Here's how the part is built. I have some questions about the finished solid (model axes, mm). Face numbers are marked on the shaded views. A direction names the side the tool comes from. Coordinates: 2 decimals unless noted, no trailing zeros. Loops run counter-clockwise (first coordinate to the right, second up) from the corner with the lowest first, then second, coordinate; pieces in that order, holes last. Notation, with made-up numbers: (65.25, 61) -> (96.25, 61) arc R26 cw to (96.25, 82) -> close; hole circle Ø7 at (-33.75, 87). An arc over 180 degrees is marked (long way). Use CSV: the item, a comma, the result in double quotes. Start each with the question number.
from build123d import *

# Parameters (mm, degrees)
BOSS_EXTRU_1_DEPTH      = 20
ENL_V_MAT_EXTRU_1_REACH = 77.705
ESQUISSE2_R             = 1.5
D_GAGEMENT_M31_D        = 3.4
D_GAGEMENT_M31_DEPTH    = 57.5
D_GAGEMENT_M31_TIP      = 1.021463052
CONG_1_R                = 10
CONG_2_R                = 5


with BuildPart() as part:
    # Esquisse1 → Boss.-Extru.1 (new body)
    with BuildSketch(Plane.XY):
        Polygon((0, 0), (4, 0), (4, 41), (53.5, 41), (53.5, 0), (57.5, 0), (57.5, 45), (0, 45), align=None)
    extrude(amount=BOSS_EXTRU_1_DEPTH)

    # Enlèv. mat.-Extru.1: up to this face of the body (flat: up to its plane)
    enl_v_mat_extru_1_end = Plane(part.part.faces().sort_by_distance((0, 22.5, 10))[0])
    # Esquisse2 → Enlèv. mat.-Extru.1 (cut, up to the picked face)
    with BuildSketch(Plane(origin=(57.5, 0, 0), x_dir=(0, 0, -1), z_dir=(1, 0, 0)), mode=Mode.PRIVATE) as enl_v_mat_extru_1_sk1:
        with Locations((-10, 5.5)):
            Circle(ESQUISSE2_R)
    enl_v_mat_extru_1_tool1 = split(extrude(enl_v_mat_extru_1_sk1.sketch, amount=-ENL_V_MAT_EXTRU_1_REACH, mode=Mode.PRIVATE), bisect_by=enl_v_mat_extru_1_end, keep=Keep.BOTH, mode=Mode.PRIVATE)
    add(enl_v_mat_extru_1_tool1.solids().sort_by(Axis((57.5, 5.5, 10), (-1, 0, 0)))[0], mode=Mode.SUBTRACT)

    # Dégagement M31
    with Locations(Plane(origin=(57.5, 0, 0), x_dir=(0, 0, -1), z_dir=(1, 0, 0))):
        with Locations((-10, 5.5)):
            Hole(D_GAGEMENT_M31_D / 2, depth=D_GAGEMENT_M31_DEPTH)
            with Locations((0, 0, -(D_GAGEMENT_M31_DEPTH + D_GAGEMENT_M31_TIP / 2))):  # 118° drill point
                Cone(0, D_GAGEMENT_M31_D / 2, D_GAGEMENT_M31_TIP, mode=Mode.SUBTRACT)

    # Congé1
    cong_1_edges = [part.edges().sort_by_distance(p)[0] for p in [
        (55.5, 0, 0),
        (55.5, 0, 20),
        (2, 0, 0),
        (2, 0, 20),
    ]]
    fillet(cong_1_edges, radius=CONG_1_R - 0.0001)  # a hair under: the kernel refuses the full size

    # Congé2
    cong_2_edges = [part.edges().sort_by_distance(p)[0] for p in [
        (0, 45, 10),
        (57.5, 45, 10),
    ]]
    fillet(cong_2_edges, radius=CONG_2_R)


solid = part.part
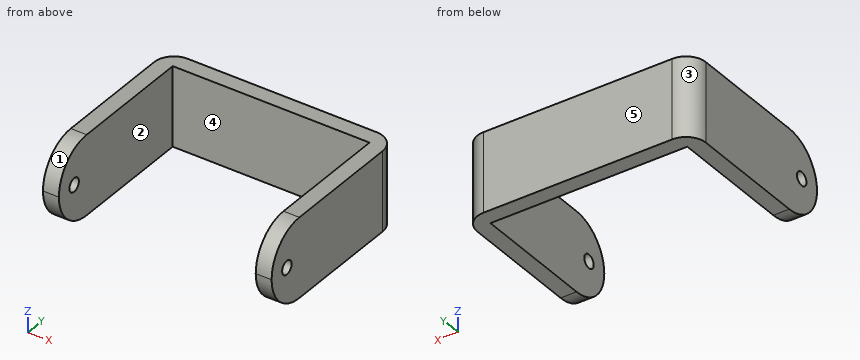
1) Please list where these lines run through material, in increasing order: L1, parallel to X at y = 18.5, z = 2.5; L2, parallel to Z at x = 1, y = 5; L3, parallel to Y at x = 35.5, z = 4.25. Write a range as [from, to].
2) Thinking about a two-plate mould opening in X: for the marked faces 1, 2 and 3, which applies, pulls with the +X half, pulls with the -X half, needs draft (parallel to the pull), parting line crosses it, or undercut?
3) I want a section at A-A, the plane y = 23. Please give me the cut outline in (x, z), plus the area to 3 significant figures.
4) I want a section at C-C, the plane y = 5.5. Please give me the cut outline in (x, z), plus the area to 3 significant figures.
5) For P1, Ø5, axis at x = 32, z = 10, coming from the -Y side; P2, Ø4, axis at x = 6.5, y = 31, coming from the -Z side; P3, Ø5.5, axis at y = 5.5, z = 10, coming from the -X side; P4, Ø12, axis at x = 8, z = 5, coming from the -Y side, each with a flat end and sliding along its axis, tell me the tip position at first contact or that it passes through.
6) I want a section at B-B, the plane z = 9.25. Please give me the cut outline in (x, y).
7) Which directions (+Z, -Z, +X, -X, +Y, -Y) give clear straight access to the entire face, cutting with the end or side of a thin tool? Please do the marked faces 4 and 5.
8) I want a section at D-D, the plane x = 8. Please give me the cut outline in (y, z), plus the area to 3 significant figures.
Return value:
1,L1,"x = [0, 4], [53.5, 57.5]"
1,L2,"z = [1.34, 8.38], [11.62, 18.66]"
1,L3,"y = [41, 45]"
2,face 1,"needs draft"
2,face 2,"undercut"
2,face 3,"pulls with the -X half"
3,outline,"(0, 0) -> (4, 0) -> (4, 20) -> (0, 20) -> close; (53.5, 0) -> (57.5, 0) -> (57.5, 20) -> (53.5, 20) -> close"
3,area,"160 mm²"
4,outline,"(0, 1.07) -> (4, 1.07) -> (4, 8.3) -> (0, 8.3) -> close; (0, 11.7) -> (4, 11.7) -> (4, 18.93) -> (0, 18.93) -> close; (53.5, 1.07) -> (57.5, 1.07) -> (57.5, 8.3) -> (53.5, 8.3) -> close; (53.5, 11.7) -> (57.5, 11.7) -> (57.5, 18.93) -> (53.5, 18.93) -> close"
4,area,"116 mm²"
5,P1,"stops at y = 41"
5,P2,"passes through"
5,P3,"stops at x = 0"
5,P4,"stops at y = 0.01"
6,outline,"(0, 0.03) -> (4, 0.03) -> (4, 3.97) -> (0, 3.97) -> close; (0, 7.03) -> (4, 7.03) -> (4, 41) -> (53.5, 41) -> (53.5, 7.03) -> (57.5, 7.03) -> (57.5, 40) arc R5 ccw to (52.5, 45) -> (5, 45) arc R5 ccw to (0, 40) -> close; (53.5, 0.03) -> (57.5, 0.03) -> (57.5, 3.97) -> (53.5, 3.97) -> close"
7,face 4,"+Z, -Z, -Y"
7,face 5,"+Z, -Z, +X, -X, +Y"
8,outline,"(41, 0) -> (45, 0) -> (45, 20) -> (41, 20) -> close"
8,area,"80.0 mm²"
